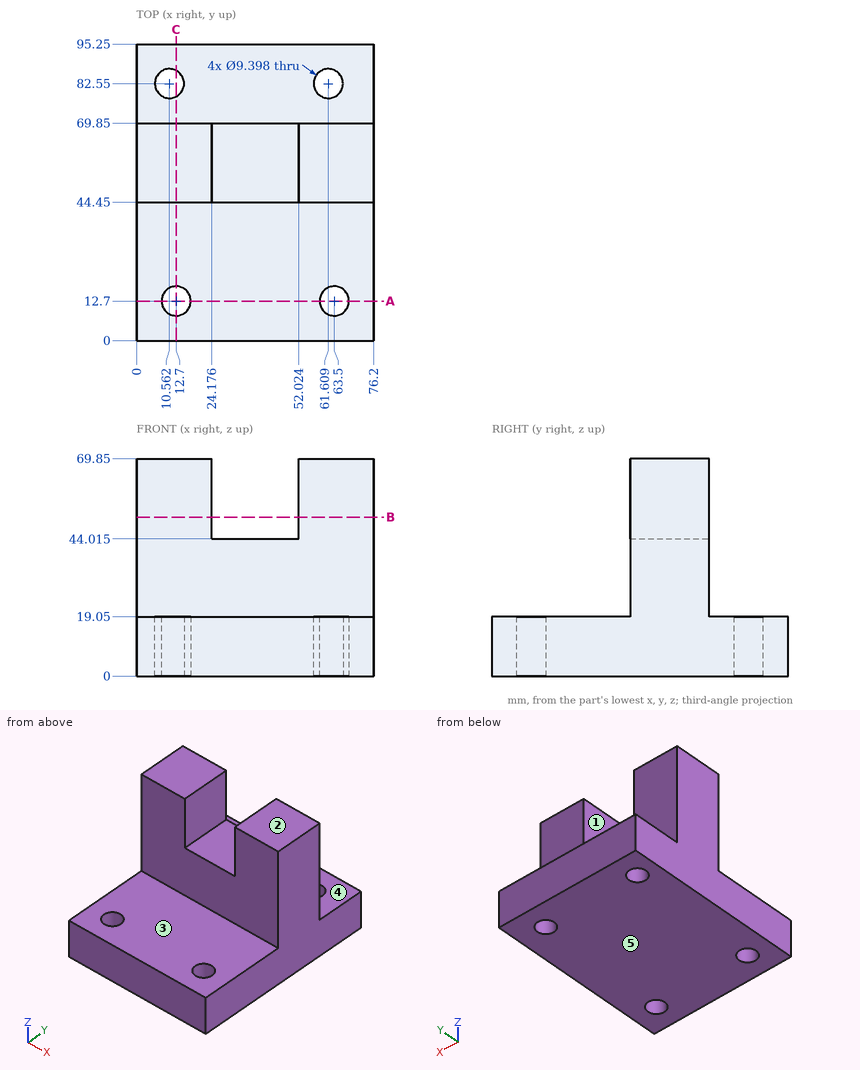
Input: dimensioned drawing with shaded views. Units: mm. Origin: part minimum x, y, z. A direction names the side the tool comes from. Coordinates: 2 decimals unless noted, no trailing zeros. Write each loop counter-clockwise with the first axis right and the second up, starting at its lowest first coordinate (ties: lowest second). Pieces come first, ordered by that corner, then holes. Notation, with made-up numbers: M 32,77 L 84,77 A23 cw 84,105 Z; hole C 60,23 d11. An arc over 180 degrees is marked long. Answer as CSV lines item,"result". Start each with the question number.
Q1. Cut plane C-C on x = 12.7. Count the separate pieces of the cut face and the enclosed holes in it, then the cut area to 3 significant figures.
Q2. Pin query (flat end, axial travel): P1, Ø12, axis at y = 77.5, z = 51, coming from the -X side; P2, Ø4, axis at x = 52, y = 34.5, coming from the +Z side. Return the tip coordinate at first contact, or that it passes through.
Q3. Cut plane B-B on z = 51. Return the cut outline in (x, y), then the cut area to 3 significant figures.
Q4. Reachability of the marked faces 1, 2, 3, 4 and 5 from +Z, -Z, +X, -X, +Y, -Y: full face, straight path, thin tool, end or side. Return the list, or none.
Q5. Line query: line 1 (X direction, y = 51, z = 56); line 2 (Y direction, x = 12, z = 6); line 3 (X direction, y = 12, z = 7). Output: solid intervals per line, ascending. Write a range as from..to.
Q6. Cut plane A-A on y = 12.7. Return the cut outline in (x, z), then the cut area to 3 significant figures.
Findings below:
1,separate pieces,"3"
1,enclosed holes,"0"
1,area,"2,770 mm2"
2,P1,"passes through"
2,P2,"stops at z = 19.05"
3,outline,"M 0,44.45 L 24.18,44.45 L 24.18,69.85 L 0,69.85 Z; M 52.02,44.45 L 76.2,44.45 L 76.2,69.85 L 52.02,69.85 Z"
3,area,"1,230 mm2"
4,face 1,"+Z, +Y, -Y"
4,face 2,"+Z, +X, -X, +Y, -Y"
4,face 3,"+Z, +X, -X, -Y"
4,face 4,"+Z, +X, -X, +Y"
4,face 5,"-Z, +X, -X, +Y, -Y"
5,line 1,"x = 0..24.18, 52.02..76.2"
5,line 2,"y = 0..8.05, 17.35..78.08, 87.02..95.25"
5,line 3,"x = 0..8.05, 17.35..58.85, 68.15..76.2"
6,outline,"M 0,0 L 8,0 L 8,19.05 L 0,19.05 Z; M 17.4,0 L 58.8,0 L 58.8,19.05 L 17.4,19.05 Z; M 68.2,0 L 76.2,0 L 76.2,19.05 L 68.2,19.05 Z"
6,area,"1,090 mm2"
